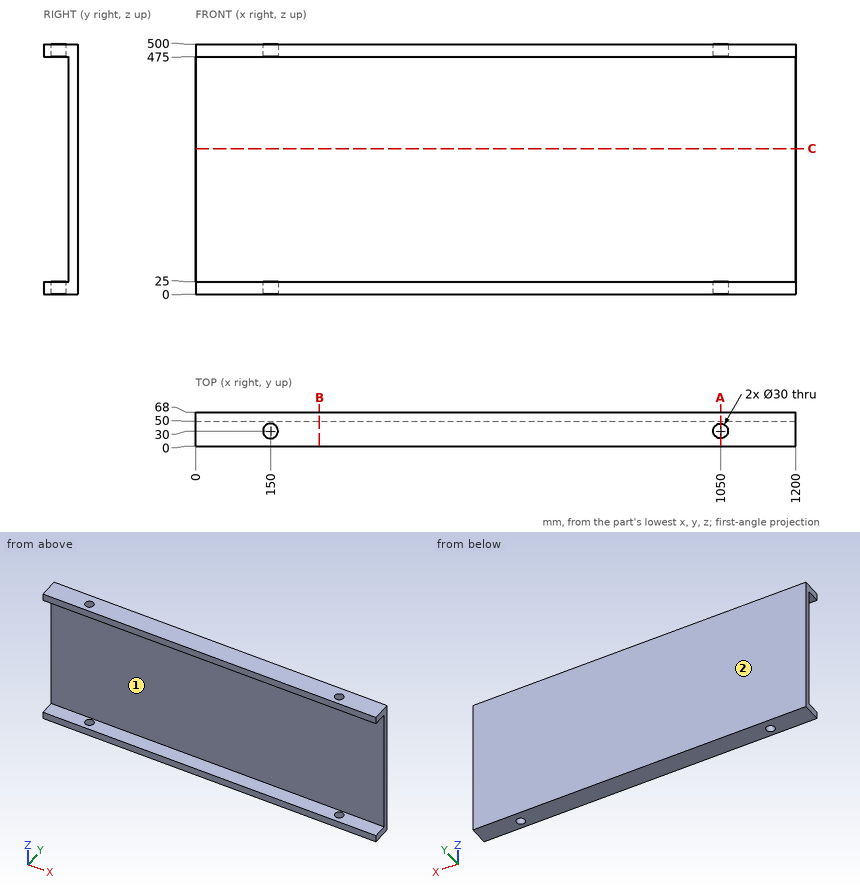
For this review, use the dimensioned drawing (mm, ordinates from the lowest corner) and the shaded views. Coordinates: 2 decimals unless noted, no trailing zeros. Order: outer loops, then holes, each group sorted by start corner. A loop starts at its lowest first (then second) coordinate and runs counter-clockwise, first axis right, second up. Notation, with made-up numbers: (-10.5, 26) - (46.5, 26) arc R23 ccw to (46.5, 54) - close; hole circle Ø3 at (-34, -24). An arc over 180 degrees is marked (long way). Answer in a Markdown table with one row per item.
(1) Consider section A-A on x = 1050. State the section outline as (y, z) points, plus the area to 3 significant figures.
Checked values:
| item | result |
|---|---|
| outline | (0, 0) - (15, 0) - (15, 25) - (0, 25) - close; (0, 475) - (15, 475) - (15, 500) - (0, 500) - close; (45, 0) - (68, 0) - (68, 500) - (45, 500) - (45, 475) - (50, 475) - (50, 25) - (45, 25) - close |
| area | 10,000 mm^2 |
(2) Consider section B-B on x = 247.5. State the section outline as (y, z) points.
Checked values:
| item | result |
|---|---|
| outline | (0, 0) - (68, 0) - (68, 500) - (0, 500) - (0, 475) - (50, 475) - (50, 25) - (0, 25) - close |
(3) Clearance check with a flat-ended pin moving along its axis: pin 1 (1 mm diameter, centred on x = 173.5, z = 120.5, fed in from -Y). State where the tip first meets the part, or that it passes through.
Checked values:
| item | result |
|---|---|
| pin 1 | y = 50 |
(4) Wall thickness on line 1 along Y through (x, z) = (1050, 13.5); line 2 along Z through (x, y) = (211, 38); line 3 along Y through (x, z) = (137.5, 342): over which ranges is each line inside the solid? List them lowest first. Write a range as from..to.
Checked values:
| item | result |
|---|---|
| line 1 | 0..15, 45..68 |
| line 2 | 0..25, 475..500 |
| line 3 | 50..68 |
(5) Consider section C-C on z = 290.5. State the section outline as (x, y) points, plus the area to 3 significant figures.
Checked values:
| item | result |
|---|---|
| outline | (0, 50) - (1200, 50) - (1200, 68) - (0, 68) - close |
| area | 21,600 mm^2 |
(6) The part is to be moulded in two halves that separate along Z. For the marked faces 1 and 2, say which applies: released by +Z, released by -Z, zero draft, split by the parting line, or undercut.
Checked values:
| item | result |
|---|---|
| face 1 | undercut |
| face 2 | zero draft |
